Geometry: final body of the model. Coordinates: model frame, mm. Face numbers are marked on the shaded views. A direction names the side the tool comes from. Coordinates: 2 decimals unless noted, no trailing zeros. Order: outer loops, then holes, each group sorted by start corner. A loop starts at its lowest first (then second) coordinate and runs counter-clockwise, first axis right, second up. Notation, with made-up numbers: M 1.25,-9.5 L 17.25,-9.5 A14 ccw 17.25,-5.5 Z; hole C 72.25,-5 d1. An arc over 180 degrees is marked long. Use CSV: the item, a comma, the result in double quotes. Start each with the question number.
Q1. Access query for the marked faces 3 and 4. Directions: +Z, -Z, +X, -X, +Y, -Y. A direction counts if a zero-diameter tool reaches every point of the face in a straight line with its end or side. Return the directions, or none.
Q2. Section query C-C, the plane x = 0. Output: boundary loops of the cut face in (y, z), and give its area (3 significant figures).
Q3. Section query B-B, the plane z = 32. Output: boundary loops of the cut face in (x, y), and give its area (3 significant figures).
Q4. Section query A-A, the plane y = -8.5. Output: boundary loops of the cut face in (x, z), and give its area (3 significant figures).
Q5. Ray query, probe 1 along Z at (x, y) = (1, -11.5); probe 2 along X at (y, z) = (-1.5, -21.5); probe 3 along Z at (x, y) = (35, -8). Return the intervals inside material, ascending.
Q6. Mould query, pull axis X, two halves, no side actions, for the marked faces 1 and 2. Classes: +X half, -X half, draft (parallel to the pull), parting line (faces both ways), or undercut.
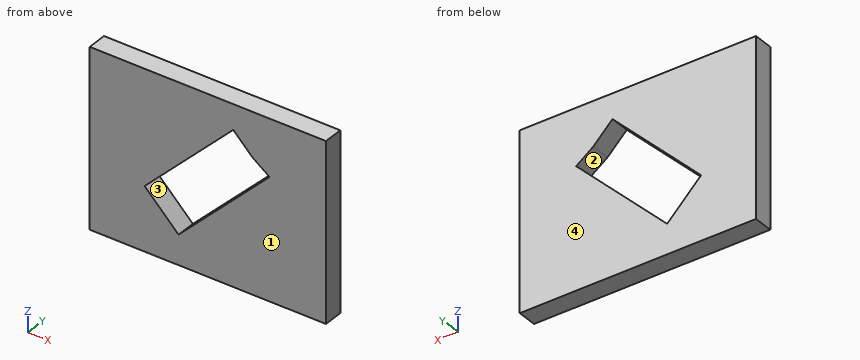
from build123d import *

# Parameters (mm, degrees)
F0_W     = 152.4
F0_H     = 114.3
F1_DEPTH = 12.7


with BuildPart() as f1:
    # F0 (on Front) → F1 (new body)
    with BuildSketch(Plane.XZ):
        with Locations((0, 0.077839)):
            Rectangle(F0_W, F0_H)
        Polygon((16.373465, 41.100174), (28.73682, 28.73682), (39.803969, 20.706104), (-18.896834, -37.994699), (-40.809121, -16.082412), align=None, mode=Mode.SUBTRACT)
    extrude(amount=F1_DEPTH)


solid = f1.part
Responses:
1,face 3,"+Y, -Y"
1,face 4,"+Z, -Z, +X, -X, +Y"
2,outline,"M -12.7,-57.07 L 0,-57.07 L 0,-19.1 L -12.7,-19.1 Z; M -12.7,24.73 L 0,24.73 L 0,57.23 L -12.7,57.23 Z"
2,area,"895 mm²"
3,outline,"M -76.2,-12.7 L 7.27,-12.7 L 7.27,0 L -76.2,0 Z; M 25.47,-12.7 L 76.2,-12.7 L 76.2,0 L 25.47,0 Z"
3,area,"1,700 mm²"
4,outline,"M -76.2,-57.07 L 76.2,-57.07 L 76.2,57.23 L -76.2,57.23 Z; hole M -40.81,-16.08 L -18.9,-37.99 L 39.8,20.71 L 28.74,28.74 L 16.37,41.1 Z"
4,area,"14,900 mm²"
5,probe 1,"z = -57.07 to -18.1, 25.73 to 57.23"
5,probe 2,"x = -76.2 to -35.39, -2.4 to 76.2"
5,probe 3,"z = -57.07 to 15.9, 24.19 to 57.23"
6,face 1,"draft"
6,face 2,"undercut"
